Check sheet for the modelled part. Datum: model origin and axes. Units: mm. A direction names the side the tool comes from. Round coordinates to 2 decimals unless told otherwise and drop trailing zeros. Loops run counter-clockwise (first coordinate to the right, second up) from the corner with the lowest first, then second, coordinate; pieces in that order, holes last. Notation, with made-up numbers: (51.25, -4.75) - (105.25, -4.75) arc R19 ccw to (105.25, 10.25) - close; hole circle Ø2 at (-2, 18.5). An arc over 180 degrees is marked (long way). Put each result on its own line as item: value.
```python
from build123d import *

# Parameters (mm, degrees)
SKETCH_1_R          = 6
SKETCH_1_R_2        = 3.05
EXTRUDE_1_DEPTH     = 25
SKETCH_2_W          = 4.705017592
SKETCH_2_H          = 2
EXTRUDE_2_DEPTH     = 12
SKETCH_4_W          = 10.5
SKETCH_4_H          = 6.5
EXTRUDE_3_DEPTH     = 25
SKETCH_6_R          = 1.5
CUT_EXTRUDE_3_DEPTH = 10
SKETCH_5_W          = 5.5
SKETCH_5_H          = 2.6
CUT_EXTRUDE_4_DEPTH = 5
CUT_EXTRUDE_8_DEPTH = 2.6
EXTRUDE_4_DEPTH     = 25
EXTRUDE_START       = 2
SKETCH_14_W         = 10.5
SKETCH_14_H         = 25
SKETCH_14_R         = 1.5
EXTRUDE_5_DEPTH     = 2
CUT_EXTRUDE_9_DEPTH = 30.391636651


with BuildPart() as part:
    # Эскиз1 → Бобышка-Вытянуть1 (new body)
    with BuildSketch(Plane(origin=(0, 0, 0), x_dir=(1, 0, 0), z_dir=(0, 1, 0))):
        with Locations(Location((0, 0, 0), (0, 0, 270))):
            Circle(SKETCH_1_R)
        with Locations(Location((0, 0, 0), (0, 0, 270))):
            Circle(SKETCH_1_R_2, mode=Mode.SUBTRACT)
    extrude(amount=EXTRUDE_1_DEPTH)

    # Эскиз2 → Бобышка-Вытянуть2 (add)
    with BuildSketch(Plane.XZ):
        with Locations((0.023466422, 3.73)):
            Rectangle(SKETCH_2_W, SKETCH_2_H)
    extrude(amount=-EXTRUDE_2_DEPTH)

    # Эскиз4 → Бобышка-Вытянуть3 (add, through all)
    with BuildSketch(Plane.XZ):
        with Locations((0, 5.98)):
            Rectangle(SKETCH_4_W, SKETCH_4_H)
    extrude(amount=-EXTRUDE_3_DEPTH)

    # Эскиз6 → Вырез-Вытянуть3 (cut)
    with BuildSketch(Plane.XY.offset(9.23)):
        with Locations((0, 5)):
            Circle(SKETCH_6_R)
    cut_extrude_3 = extrude(amount=-CUT_EXTRUDE_3_DEPTH, mode=Mode.SUBTRACT)

    # Эскиз5 → Вырез-Вытянуть4 (cut)
    with BuildSketch(Plane.XZ):
        with Locations((0, 6.03)):
            Rectangle(SKETCH_5_W, SKETCH_5_H)
    cut_extrude_4 = extrude(amount=-CUT_EXTRUDE_4_DEPTH, mode=Mode.SUBTRACT)

    # Эскиз11 → Вырез-Вытянуть8 (cut)
    with BuildSketch(Plane(origin=(0, 0, 7.33), x_dir=(-1, 0, 0), z_dir=(0, 0, -1))):
        Polygon((-2.75, 6.58771324), (-2.75, 7.08771324), (0, 8.675426481), (2.75, 7.08771324), (2.75, 6.58771324), (2.75, 3.41228676), (0, 1.824573519), (-2.75, 3.41228676), align=None)
    cut_extrude_8 = extrude(amount=CUT_EXTRUDE_8_DEPTH, mode=Mode.SUBTRACT)

    # Зеркальное отражение1: Вырез-Вытянуть3, Вырез-Вытянуть4, Вырез-Вытянуть8 across plane
    add(cut_extrude_3.mirror(Plane(origin=(0, 12.5, 0), x_dir=(0, 0, 1), z_dir=(0, -1, 0))), mode=Mode.SUBTRACT)
    add(cut_extrude_4.mirror(Plane(origin=(0, 12.5, 0), x_dir=(0, 0, 1), z_dir=(0, -1, 0))), mode=Mode.SUBTRACT)
    add(cut_extrude_8.mirror(Plane(origin=(0, 12.5, 0), x_dir=(0, 0, 1), z_dir=(0, -1, 0))), mode=Mode.SUBTRACT)

    # Эскиз13 → Бобышка-Вытянуть4 (add, through all)
    with BuildSketch(Plane(origin=(0, 25, 0), x_dir=(1, 0, 0), z_dir=(0, 1, 0))):
        with BuildLine():
            Line((-5.25, -2.90473751), (-5.25, -9.23))
            ThreePointArc((-5.25, -9.23), (0, 10.618634564), (5.25, -9.23))
            Line((5.25, -9.23), (5.25, -2.90473751))
            ThreePointArc((5.25, -2.90473751), (0, 6), (-5.25, -2.90473751))
        make_face()
    extrude(amount=-EXTRUDE_4_DEPTH)

    # Эскиз14 → Бобышка-Вытянуть5 (add)
    with BuildSketch(Plane.XY.offset(9.23).offset(EXTRUDE_START)):
        with Locations((0, 12.5)):
            Rectangle(SKETCH_14_W, SKETCH_14_H)
        with Locations((0, 20)):
            Circle(SKETCH_14_R, mode=Mode.SUBTRACT)
        with Locations((0, 5)):
            Circle(SKETCH_14_R, mode=Mode.SUBTRACT)
    extrude(amount=-EXTRUDE_5_DEPTH)

    # Эскиз15 → Вырез-Вытянуть9 (cut, through all)
    with BuildSketch(Plane.XZ):
        with BuildLine():
            Line((-5.25, 9.23), (-5.25, 7.310095759))
            ThreePointArc((-5.25, 7.310095759), (0, -9), (5.25, 7.310095759))
            Line((5.25, 7.310095759), (5.25, 9.23))
            ThreePointArc((5.25, 9.23), (0, -10.618634564), (-5.25, 9.23))
        make_face()
    extrude(amount=-CUT_EXTRUDE_9_DEPTH, mode=Mode.SUBTRACT)

    # Фаска1
    # the kernel refuses this chamfer: 4.36872896, 1 mm, written as the material it adds along each edge
    with BuildSketch(Plane(origin=(-5.25, 0, 7.310095759), x_dir=(0.003980651580542702, 0, 0.9999920771751115), z_dir=(0, 1, 0))) as chamfer_1_piece_1_section:
        with BuildLine():
            Line((4.499702082, 0), (-0.54914754, -0.499943041))
            Line((-0.54914754, -0.499943041), (-0.616269571, -0.444006022))
            ThreePointArc((-0.616269571, -0.444006022), (-0.289511406, -0.238197361), (-0.070765054, 0.051250602))
            Line((-0.070765054, 0.051250602), (0.000347808, 0.087373887))
            ThreePointArc((0.000347808, 0.087373887), (2.250163198, 0.078418085), (4.50004989, 0.087373887))
            Line((4.50004989, 0.087373887), (4.499702082, 0))
        make_face()
    chamfer_1_piece_1 = extrude(amount=25, mode=Mode.PRIVATE)
    chamfer_1_piece_1 = split(chamfer_1_piece_1, bisect_by=Plane(origin=(-5.368726711, 12.5, 11.23), z_dir=(0, 0, -1)), keep=Keep.TOP, mode=Mode.PRIVATE)
    add(chamfer_1_piece_1)

    # Фаска2
    # the kernel refuses this chamfer: 4.36872896, 1 mm, written as the material it adds along each edge
    with BuildSketch(Plane(origin=(5.25, 0, 7.310095759), x_dir=(-0.0039806515805427085, 0, 0.9999920771751115), z_dir=(0, 1, 0))) as chamfer_2_piece_1_section:
        with BuildLine():
            Line((4.499702082, 0), (-0.54914754, 0.499943041))
            Line((-0.54914754, 0.499943041), (-0.616269571, 0.444006022))
            ThreePointArc((-0.616269571, 0.444006022), (-0.289511406, 0.238197361), (-0.070765054, -0.051250602))
            Line((-0.070765054, -0.051250602), (0.000347808, -0.087373887))
            ThreePointArc((0.000347808, -0.087373887), (2.250163198, -0.078418085), (4.50004989, -0.087373887))
            Line((4.50004989, -0.087373887), (4.499702082, 0))
        make_face()
    chamfer_2_piece_1 = extrude(amount=25, mode=Mode.PRIVATE)
    chamfer_2_piece_1 = split(chamfer_2_piece_1, bisect_by=Plane(origin=(5.368726711, 12.5, 11.23), z_dir=(0, 0, -1)), keep=Keep.TOP, mode=Mode.PRIVATE)
    add(chamfer_2_piece_1)


solid = part.part
```
Item 1: Release check for a two-part mould opening along X. For faces 1 (the cylindrical face through (0, 12, -9)), 2 (the flat face through (0, 3, 7.33)), 3 (the flat face through (0, 13, 11.23)) record: +X half, -X half, draft (parallel to the pull), parting line (faces both ways), or undercut.
Filled sheet:
face 1: parting line
face 2: undercut
face 3: draft
Item 2: Thickness scan on line 1 (Y direction, x = 0, z = 4.25); line 2 (Z direction, x = 0.25, y = 3); line 3 (X direction, y = 19, z = 0). Record the ranges inside material, lowest first. Write a range as from..to.
Filled sheet:
line 1: 0..3.5, 6.5..18.5, 21.5..25
line 2: -9..-3.04, 2.73..4.73, 7.33..11.23
line 3: -9..-3.05, 3.05..9
Item 3: Section check C-C on y = 9. Enter the section's corners in (x, z).
Filled sheet:
outline: (-5.73, 6.94) arc R9 ccw (long way) to (5.73, 6.94) - (5.29, 11.23) - (-5.29, 11.23) - close; hole (-1.36, 2.73) arc R3.05 ccw (long way) to (1.36, 2.73) - close
Item 4: Section check B-B on z = 0. Enter the section's corners in (x, y).
Filled sheet:
outline: (-9, 0) - (-3.05, 0) - (-3.05, 25) - (-9, 25) - close; (3.05, 0) - (9, 0) - (9, 25) - (3.05, 25) - close
Item 5: Section check A-A on y = 22. Enter the section's corners in (x, z), then the cut area to 3 significant figures.
Filled sheet:
outline: (-5.73, 6.94) arc R9 ccw (long way) to (5.73, 6.94) - (5.29, 11.23) - (-5.29, 11.23) - close; hole (-2.75, 4.73) - (2.75, 4.73) - (2.75, 7.33) - (-2.75, 7.33) - close; hole (-1.36, 2.73) arc R3.05 ccw (long way) to (1.36, 2.73) - close
area: 243 mm²
Item 6: Go/stop test with flat-tipped pins: pin 1 (6 mm diameter, centred on x = 0, y = 6, fed in from +Z); pin 2 (1.5 mm diameter, centred on y = 7, z = -7, fed in from +X); pin 3 (2 mm diameter, centred on y = 22.5, z = 6.5, fed in from +X); pin 4 (3 mm diameter, centred on x = -6.5, y = 17, fed in from -Z). Record where each tip stops, or that it passes through.
Filled sheet:
pin 1: z = 11.23
pin 2: x = 6.48
pin 3: x = 7.12
pin 4: z = -7.48
Item 7: Section check D-D on z = 8.75. Enter the section's corners in (x, y).
Filled sheet:
outline: (-5.55, 0) - (5.55, 0) - (5.55, 25) - (-5.55, 25) - close; hole circle Ø3 at (0, 5); hole circle Ø3 at (0, 20)
Item 8: Tool access check on faces 4 (the flat face through (-2.75, 3, 6)), 5 (the flat face through (1.394, 17.13, 6.048)), 6 (the flat face through (0, 23, 2.73)), 7 (the cylindrical face through (-0.195, 18.513, 3.707)). Record the directions out of +Z, -Z, +X, -X, +Y, -Y that give a thin tool (end or side, any length) a straight path to the whole face; none if there is none.
Filled sheet:
face 4: -Y
face 5: +Y
face 6: +Y, -Y
face 7: +Z
